Part model, mm, in its own coordinate system. A direction names the side the tool comes from. Give positions to 0.01 mm unless a question says otherwise; leave off trailing zeros. Write each loop counter-clockwise with the first axis right and the second up, starting at its lowest first coordinate (ties: lowest second). Pieces come first, ordered by that corner, then holes.
```python
from build123d import *

# Parameters (mm, degrees)
SKETCH1_R           = 2.2098
BOSS_EXTRUDE1_DEPTH = 3.175
SKETCH2_R           = 3.1623
CUT_EXTRUDE3_DEPTH  = 1.27
SKETCH3_R           = 2.2098
BOSS_EXTRUDE2_DEPTH = 1.253000034


with BuildPart() as part:
    # Sketch1 → Boss-Extrude1 (new body)
    with BuildSketch(Plane.XY):
        with BuildLine():
            Line((-50.8, -31.75), (50.8, -31.75))
            ThreePointArc((50.8, -31.75), (55.290128061, -29.890128061), (57.15, -25.4))
            Line((57.15, -25.4), (57.15, 25.4))
            ThreePointArc((57.15, 25.4), (55.290128061, 29.890128061), (50.8, 31.75))
            Line((50.8, 31.75), (-50.8, 31.75))
            ThreePointArc((-50.8, 31.75), (-55.290128061, 29.890128061), (-57.15, 25.4))
            Line((-57.15, 25.4), (-57.15, -25.4))
            ThreePointArc((-57.15, -25.4), (-55.290128061, -29.890128061), (-50.8, -31.75))
        make_face()
        with Locations((-50.8, -25.4)):
            Circle(SKETCH1_R, mode=Mode.SUBTRACT)
        with Locations((-38.1, -25.4)):
            Circle(SKETCH1_R, mode=Mode.SUBTRACT)
        with Locations(Location((-50.8, 25.4, 0), (0, 0, 180))):
            Circle(SKETCH1_R, mode=Mode.SUBTRACT)
        with Locations(Location((-38.1, 25.4, 0), (0, 0, 180))):
            Circle(SKETCH1_R, mode=Mode.SUBTRACT)
        with Locations((50.8, 25.4)):
            Circle(SKETCH1_R, mode=Mode.SUBTRACT)
        with Locations((38.1, 25.4)):
            Circle(SKETCH1_R, mode=Mode.SUBTRACT)
        with Locations(Location((50.8, -25.4, 0), (0, 0, 180))):
            Circle(SKETCH1_R, mode=Mode.SUBTRACT)
        with Locations(Location((38.1, -25.4, 0), (0, 0, 180))):
            Circle(SKETCH1_R, mode=Mode.SUBTRACT)
    extrude(amount=-BOSS_EXTRUDE1_DEPTH)

    # Sketch2 → Cut-Extrude3 (cut)
    with BuildSketch(Plane.XY):
        with BuildLine():
            Line((50.8, 30.7975), (-50.8, 30.7975))
            ThreePointArc((-50.8, 30.7975), (-54.616608851, 29.216608851), (-56.1975, 25.4))
            Line((-56.1975, 25.4), (-56.1975, -25.4))
            ThreePointArc((-56.1975, -25.4), (-54.616608851, -29.216608851), (-50.8, -30.7975))
            Line((-50.8, -30.7975), (50.8, -30.7975))
            ThreePointArc((50.8, -30.7975), (54.616608851, -29.216608851), (56.1975, -25.4))
            Line((56.1975, -25.4), (56.1975, 25.4))
            ThreePointArc((56.1975, 25.4), (54.616608851, 29.216608851), (50.8, 30.7975))
        make_face()
        with Locations((38.1, 25.4)):
            Circle(SKETCH2_R, mode=Mode.SUBTRACT)
        with Locations((50.8, 25.4)):
            Circle(SKETCH2_R, mode=Mode.SUBTRACT)
        with Locations((50.8, -25.4)):
            Circle(SKETCH2_R, mode=Mode.SUBTRACT)
        with Locations((38.1, -25.4)):
            Circle(SKETCH2_R, mode=Mode.SUBTRACT)
        with Locations((-38.1, -25.4)):
            Circle(SKETCH2_R, mode=Mode.SUBTRACT)
        with Locations((-50.8, -25.4)):
            Circle(SKETCH2_R, mode=Mode.SUBTRACT)
        with Locations((-38.1, 25.4)):
            Circle(SKETCH2_R, mode=Mode.SUBTRACT)
        with Locations((-50.8, 25.4)):
            Circle(SKETCH2_R, mode=Mode.SUBTRACT)
    extrude(amount=-CUT_EXTRUDE3_DEPTH, mode=Mode.SUBTRACT)

    # Sketch3 → Boss-Extrude2 (add)
    with BuildSketch(Plane(origin=(0, 0, -3.175), x_dir=(-1, 0, 0), z_dir=(0, 0, -1))):
        with BuildLine():
            Line((-57.15, 25.4), (-57.15, -25.4))
            ThreePointArc((-57.15, -25.4), (-55.290128061, -29.890128061), (-50.8, -31.75))
            Line((-50.8, -31.75), (50.8, -31.75))
            ThreePointArc((50.8, -31.75), (55.290128061, -29.890128061), (57.15, -25.4))
            Line((57.15, -25.4), (57.15, 25.4))
            ThreePointArc((57.15, 25.4), (55.290128061, 29.890128061), (50.8, 31.75))
            Line((50.8, 31.75), (-50.8, 31.75))
            ThreePointArc((-50.8, 31.75), (-55.290128061, 29.890128061), (-57.15, 25.4))
        make_face()
        with Locations((-50.8, -25.4)):
            Circle(SKETCH3_R, mode=Mode.SUBTRACT)
        with Locations((-38.1, -25.4)):
            Circle(SKETCH3_R, mode=Mode.SUBTRACT)
        with Locations(Location((38.1, -25.4, 0), (0, 0, 180))):
            Circle(SKETCH3_R, mode=Mode.SUBTRACT)
        with Locations(Location((50.8, -25.4, 0), (0, 0, 180))):
            Circle(SKETCH3_R, mode=Mode.SUBTRACT)
        with Locations((50.8, 25.4)):
            Circle(SKETCH3_R, mode=Mode.SUBTRACT)
        with Locations((38.1, 25.4)):
            Circle(SKETCH3_R, mode=Mode.SUBTRACT)
        with Locations(Location((-38.1, 25.4, 0), (0, 0, 180))):
            Circle(SKETCH3_R, mode=Mode.SUBTRACT)
        with Locations(Location((-50.8, 25.4, 0), (0, 0, 180))):
            Circle(SKETCH3_R, mode=Mode.SUBTRACT)
    extrude(amount=BOSS_EXTRUDE2_DEPTH)


solid = part.part
```
1) Saw through at B-B, the plane y = 7. Write the cut outline in (x, z), then the cut area to 3 significant figures.
Answers follow:
outline: (-57.15, -4.43) - (57.15, -4.43) - (57.15, 0) - (56.2, 0) - (56.2, -1.27) - (-56.2, -1.27) - (-56.2, 0) - (-57.15, 0) - close
area: 363 mm2
2) Saw through at C-C, the plane z = -2. Count the separate pieces of the cut face and the enclosed holes in it, then the cut area to 3 significant figures.
Answers follow:
separate pieces: 1
enclosed holes: 8
area: 7,100 mm2
3) Saw through at A-A, the plane x = 38.1. Write the cut outline in (y, z).
Answers follow:
outline: (-31.75, -4.43) - (-27.61, -4.43) - (-27.61, 0) - (-28.56, 0) - (-28.56, -1.27) - (-30.8, -1.27) - (-30.8, 0) - (-31.75, 0) - close; (-23.19, -4.43) - (23.19, -4.43) - (23.19, 0) - (22.24, 0) - (22.24, -1.27) - (-22.24, -1.27) - (-22.24, 0) - (-23.19, 0) - close; (27.61, -4.43) - (31.75, -4.43) - (31.75, 0) - (30.8, 0) - (30.8, -1.27) - (28.56, -1.27) - (28.56, 0) - (27.61, 0) - close
4) Saw through at D-D, the plane x = -20.5. Write the cut outline in (y, z), then the cut area to 3 significant figures.
Answers follow:
outline: (-31.75, -4.43) - (31.75, -4.43) - (31.75, 0) - (30.8, 0) - (30.8, -1.27) - (-30.8, -1.27) - (-30.8, 0) - (-31.75, 0) - close
area: 203 mm2
5) Two-plate mould, pull along X, no slides. Class faces 1 (the face through (54.57, -29.26, -0.63)), 2 (the face through (-37, -23, 0)), 3 (the face through (-55.24, -29.94, -2.18)): +X half, -X half, draft (parallel to the pull), parting line (faces both ways), or undercut.
Answers follow:
face 1: undercut
face 2: draft
face 3: -X half
6) 3-axis set-ups, long thin cutter, end or side, ignore diameter. For faces 4 (the face through (48.291, 23.476, -0.626)), 5 (the face through (51, -23, 0)): which of +Z, -Z, +X, -X, +Y, -Y reach the whole face in a straight line?
Answers follow:
face 4: +Z
face 5: +Z, +X, -X, +Y, -Y
7) Wall check: L1, parallel to Y at x = -38.1, z = -2; L2, parallel to X at y = 25.4, z = -3.9; L3, parallel to X at y = -16, z = -1.15. Give the ranges that are in metal, low to high.
Answers follow:
L1: y = -31.75 to -27.61, -23.19 to 23.19, 27.61 to 31.75
L2: x = -57.15 to -53.01, -48.59 to -40.31, -35.89 to 35.89, 40.31 to 48.59, 53.01 to 57.15
L3: x = -57.15 to -56.2, 56.2 to 57.15
8) Pin check, flat tips, straight feed: pin 1 Ø5 at (x, y) = (-50.8, 25.4) entering from +Z; pin 2 Ø10 at (x, y) = (15, 23) entering from +Z. Stop position of each tip, or through.
Answers follow:
pin 1: stops at z = 0
pin 2: stops at z = -1.27
